Can you work these out from the model? Positions are in its coordinate system, mm. Face numbers are marked on the shaded views. A direction names the side the tool comes from. Round coordinates to 2 decimals unless told otherwise and drop trailing zeros. Order: outer loops, then holes, each group sorted by start corner. A loop starts at its lowest first (then second) coordinate and runs counter-clockwise, first axis right, second up.
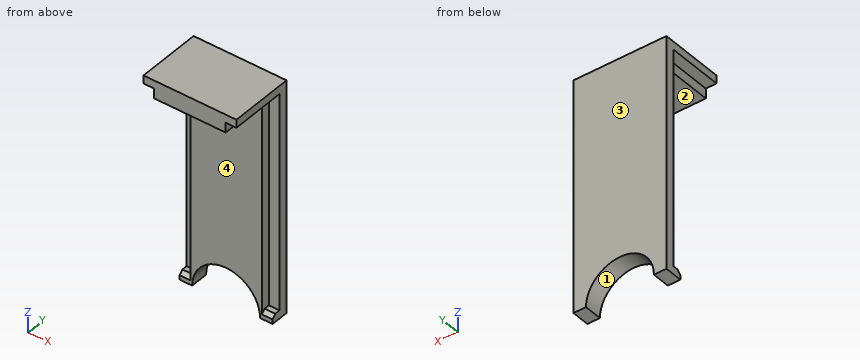
Autodesk Inventor part; units mm, degrees
ref_plane "YZ Plane" through (0, 0, 0) normal (1, 0, 0) x (0, 1, 0)
ref_plane "XZ Plane" through (0, 0, 0) normal (0, 1, 0) x (-1, 0, 0)
ref_plane "XY Plane" through (0, 0, 0) normal (0, 0, 1) x (1, 0, 0)
sketch "Sketch3" plane through (0, 0, 0) normal (0, 1, 0) x (-1, 0, 0)
  line L0 (13, 0) -> (-13, 0)
  line L1 (-13, 0) -> (-13, -65)
  line L2 (-13, -65) -> (13, -65)
  line L3 (13, -65) -> (13, 0)
  point P0 (0, 0)
  dimension "d8" = 26
  dimension "d9" = 13
  dimension "d18" = 65
extrude "Extrusion3" add sketch "Sketch3" along normal blind 5
sketch "Sketch4" plane through (0, 0, 0) normal (0, -1, 0) x (1, 0, 0)
  line L0 (-13, 0) -> (13, 0)
  line L1 (-13, -65) -> (-13, 0)
  line L2 (13, -65) -> (-13, -65)
  line L3 (13, 0) -> (13, -65)
  line L4 (13, 0) -> (-13, 0)
  line L5 (-13, 0) -> (-13, -5)
  line L6 (-13, -5) -> (13, -5)
  line L7 (13, -5) -> (13, 0)
  point P0 (0, 0)
  dimension "d14" = 5
extrude "Extrusion4" add sketch "Sketch4" along normal blind 13 contours L0 L3 L6 L1
sketch "Sketch6" plane through (0, 5, 0) normal (0, 1, 0) x (1, 0, 0)
  line L0 (-13, 0) -> (13, 0)
  line L1 (13, 0) -> (13, 65)
  line L2 (13, 65) -> (-13, 65)
  line L3 (-13, 65) -> (-13, 0)
  circle A0 centre (0, 65) radius 9.5
  point P0 (0, 0)
  dimension "d25" = 19
  dimension "d26" = 0
extrude "Extrusion6" cut sketch "Sketch6" against normal through all contours A0 L2 | L2 A0
sketch "Sketch7" plane through (13, 0, -65) normal (1, 0, 0) x (0, 0, -1)
  line L0 (-60, 0) -> (0, 0)
  line L1 (0, 0) -> (0, 5)
  line L2 (-65, 5) -> (0, 5)
  line L3 (-65, -13) -> (-65, 5)
  line L4 (-60, -13) -> (-65, -13)
  line L5 (-60, 0) -> (-60, -13)
  line L6 (-60, -13) -> (-62.75, -13)
  line L7 (-62.75, -13) -> (-62.75, 0)
  line L8 (-62.75, 0) -> (-60, 0)
  line L9 (-60, 0) -> (-60, -13)
  line L10 (-62.75, 0) -> (-2.25, 0)
  line L11 (-2.25, 0) -> (-2.25, 2.5)
  line L12 (-2.25, 2.5) -> (-62.75, 2.5)
  line L13 (-62.75, 2.5) -> (-62.75, 0)
  point P0 (-65, 0)
  dimension "d29" = 2.75
  dimension "d30" = 2.5
  dimension "d31" = 2.25
extrude "Extrusion7" cut sketch "Sketch7" against normal blind 3 contours L8 L13 L12 L11 L0 | L5 L4 L7 L8
mirror "Mirror2" about plane through (0, 0, 0) normal (1, 0, 0) of "Extrusion7"
chamfer "Chamfer1" distance 1 angle 45 2 edges at (11.5, 0, -62.75) (-11.5, 0, -62.75)
properties part number "Roof Clip"
(1) I want a section at C-C, the plane y = -7.75. List the corners of the cut face in (x, z) for me.
(2) I want a section at B-B, the plane z = -42. List the corners of the cut face in (x, y) for me, plus the area to 3 significant figures.
(3) I'm going to push flat-ended pins straight in: pin 1 Ø1.5 at (x, z) = (-0.5, -7) entering from -Y; pin 2 Ø0.9 at (x, z) = (11.5, -34.5) entering from -Y; pin 3 Ø1.5 at (x, y) = (11, -7) entering from -Z. Where does each tip first touch, or does it pass through?
(4) I want a section at D-D, the plane x = 11. List the corners of the cut face in (y, z) for me.
(5) On a 3-axis mill with a long thin cutter (end or side, diameter ignored), from which of +Z, -Z, +X, -X, +Y, -Y can I reach the whole of each face in a straight line? I mean the marked faces 3 and 4. Say none if no direction works.
(6) If we mould it in two halves opening along X, with no side actions, what happens to the marked faces 1 and 2? For each: pulls with the +X half, pulls with the -X half, needs draft (parallel to the pull), parting line crosses it, or undercut.
(7) I want a section at A-A, the plane x = 0. List the corners of the cut face in (y, z) for me, plus the area to 4 significant figures.
(8) Please list where these lines run through material, in increasing order: probe 1 along Z at (x, y) = (11.5, 2); probe 2 along Z at (x, y) = (12, -7); probe 3 along Y at (x, z) = (10.75, -19).
Ans:
1. outline: (-13, -2.25) - (-10, -2.25) - (-10, -5) - (10, -5) - (10, -2.25) - (13, -2.25) - (13, 0) - (-13, 0) - close
2. outline: (-13, 2.5) - (-10, 2.5) - (-10, 0) - (10, 0) - (10, 2.5) - (13, 2.5) - (13, 5) - (-13, 5) - close
2. area: 115 mm2
3. pin 1: stops at y = 0
3. pin 2: stops at y = 2.5
3. pin 3: stops at z = -2.25
4. outline: (-13, -2.25) - (2.5, -2.25) - (2.5, -62.75) - (1, -62.75) - (0, -63.75) - (0, -65) - (5, -65) - (5, 0) - (-13, 0) - close
5. face 3: +Z, -Z, +X, -X, +Y
5. face 4: -Z, +X, -X, -Y
6. face 1: undercut
6. face 2: needs draft
7. outline: (-13, -5) - (0, -5) - (0, -55.5) - (5, -55.5) - (5, 0) - (-13, 0) - close
7. area: 342.5 mm2
8. probe 1: z = -65 to -62.75, -2.25 to 0
8. probe 2: z = -2.25 to 0
8. probe 3: y = 2.5 to 5
